Geometry check sheet. Reference: the model listing, model coordinates, mm. A direction names the side the tool comes from. Round coordinates to 2 decimals unless told otherwise and drop trailing zeros. Order: outer loops, then holes, each group sorted by start corner. A loop starts at its lowest first (then second) coordinate and runs counter-clockwise, first axis right, second up. Notation, with made-up numbers: (8.5, 58.5) - (40.5, 58.5) arc R28 cw to (40.5, 86.5) - close; hole circle Ø8 at (-37.5, -3.5). An arc over 180 degrees is marked (long way). Return JSON: item names as keys, results as strings. Group by question number.
Q1. Gauge pin test, flat ends, axial feed: pin 1 Ø8 at (x, y) = (69.28, -40) entering from -Z; pin 2 Ø10 at (x, y) = (11, 59) entering from -Z; pin 3 Ø3 at (x, z) = (-66.5, 2.5) entering from +Y; pin 4 Ø4 at (y, z) = (3.5, 6) entering from -X. Record the tip position at first contact, or that the pin passes through.
Q2. Tool access check on faces 4 (the flat face through (55.568, -10.884, 4.93)), 5 (the cylindrical face through (60.1, -26.1, 4.9)). Record the directions out of +Z, -Z, +X, -X, +Y, -Y that give a thin tool (end or side, any length) a straight path to the whole face; none if there is none.
Q3. Sectioned sample at C-C, the plane z = 5.5. Give the number of separate pieces and of enclosed holes in the cut face, then the cut area to 3 significant figures.
Q4. Sectioned sample at A-A, the plane x = 0. Record the cut outline in (y, z), then the cut area to 3 significant figures.
Q5. Draft check along Y on faces 1 (the cylindrical face through (-82.12, -47.76, 4.93)), 2 (the cylindrical face through (0, 65, 5)), 3 (the flat face through (37.933, -42.989, 4.93)). Enter one of: pulls with the +Y half, pulls with the -Y half, needs draft (parallel to the pull), parting line crosses it, or undercut.
Q6. Sectioned sample at B-B, the plane y = 80. Record the cut outline in (x, z), then the cut area to 3 significant figures.
Q7. Material ranges on line 1 along Y through (x, z) = (0, 4); line 2 along X through (y, z) = (-43.5, 1); line 3 along X through (y, z) = (-8, 8), recorded low to high.
Q8. Sectioned sample at D-D, the plane x = 43.5. Record the cut outline in (y, z), then the cut area to 3 significant figures.
```python
from build123d import *

# Parameters (mm, degrees)
SKETCH1_R           = 5
SKETCH1_R_2         = 10
BOSS_EXTRUDE1_DEPTH = 10


with BuildPart() as part:
    # Sketch1 → Boss-Extrude1 (new body)
    with BuildSketch(Plane.XY):
        with BuildLine():
            ThreePointArc((-33.454782287, 5.779804226), (-25.528470868, 14.738869527), (-21.732848432, 26.082789225))
            Line((-21.732848432, 26.082789225), (-14.888192275, 81.828040151))
            ThreePointArc((-14.888192275, 81.828040151), (0, 95), (14.888192275, 81.828040151))
            Line((14.888192275, 81.828040151), (21.732848432, 26.082789225))
            ThreePointArc((21.732848432, 26.082789225), (25.528470868, 14.738869527), (33.454782287, 5.779804226))
            Line((33.454782287, 5.779804226), (78.30925765, -28.020467349))
            ThreePointArc((78.30925765, -28.020467349), (82.27241336, -47.5), (63.421065375, -53.807572802))
            Line((63.421065375, -53.807572802), (11.721933855, -31.862593451))
            ThreePointArc((11.721933855, -31.862593451), (0, -29.477739055), (-11.721933855, -31.862593451))
            Line((-11.721933855, -31.862593451), (-63.421065375, -53.807572802))
            ThreePointArc((-63.421065375, -53.807572802), (-82.27241336, -47.5), (-78.30925765, -28.020467349))
            Line((-78.30925765, -28.020467349), (-33.454782287, 5.779804226))
        make_face()
        with Locations((-69.282032303, -40)):
            Circle(SKETCH1_R, mode=Mode.SUBTRACT)
        with Locations((69.282032303, -40)):
            Circle(SKETCH1_R, mode=Mode.SUBTRACT)
        with Locations((0, 80)):
            Circle(SKETCH1_R, mode=Mode.SUBTRACT)
        Circle(SKETCH1_R_2, mode=Mode.SUBTRACT)
        with BuildLine():
            ThreePointArc((-4.155876324, 65.587203881), (-7.469391302, 65.0809662), (-9.234294617, 62.231268956))
            Line((-9.234294617, 62.231268956), (-13.739592483, 25.538562373))
            ThreePointArc((-13.739592483, 25.538562373), (-11.624113874, 20.196928868), (-5.987935057, 19.082574086))
            ThreePointArc((-5.987935057, 19.082574086), (0, 20), (5.987935057, 19.082574086))
            ThreePointArc((5.987935057, 19.082574086), (11.624113874, 20.196928868), (13.739592483, 25.538562373))
            Line((13.739592483, 25.538562373), (9.234294617, 62.231268956))
            ThreePointArc((9.234294617, 62.231268956), (7.469391302, 65.0809662), (4.155876324, 65.587203881))
            ThreePointArc((4.155876324, 65.587203881), (0, 65), (-4.155876324, 65.587203881))
        make_face(mode=Mode.SUBTRACT)
        with BuildLine():
            ThreePointArc((58.878122886, -29.194507469), (60.096465683, -26.071800482), (58.511007134, -23.118500753))
            Line((58.511007134, -23.118500753), (28.986840033, -0.870445058))
            ThreePointArc((28.986840033, -0.870445058), (23.303110415, -0.031686522), (19.519961457, -4.355583168))
            ThreePointArc((19.519961457, -4.355583168), (17.320508076, -10), (13.5320264, -14.726990918))
            ThreePointArc((13.5320264, -14.726990918), (11.678996541, -20.165242346), (15.247247549, -24.668117315))
            Line((15.247247549, -24.668117315), (49.276712517, -39.112768202))
            ThreePointArc((49.276712517, -39.112768202), (52.627074381, -39.009165718), (54.722246562, -36.392696412))
            ThreePointArc((54.722246562, -36.392696412), (56.291651246, -32.5), (58.878122886, -29.194507469))
        make_face(mode=Mode.SUBTRACT)
        with BuildLine():
            ThreePointArc((-54.722246562, -36.392696412), (-52.627074381, -39.009165718), (-49.276712517, -39.112768202))
            Line((-49.276712517, -39.112768202), (-15.247247549, -24.668117315))
            ThreePointArc((-15.247247549, -24.668117315), (-11.678996541, -20.165242346), (-13.5320264, -14.726990918))
            ThreePointArc((-13.5320264, -14.726990918), (-17.320508076, -10), (-19.519961457, -4.355583168))
            ThreePointArc((-19.519961457, -4.355583168), (-23.303110415, -0.031686522), (-28.986840033, -0.870445058))
            Line((-28.986840033, -0.870445058), (-58.511007134, -23.118500753))
            ThreePointArc((-58.511007134, -23.118500753), (-60.096465683, -26.071800482), (-58.878122886, -29.194507469))
            ThreePointArc((-58.878122886, -29.194507469), (-56.291651246, -32.5), (-54.722246562, -36.392696412))
        make_face(mode=Mode.SUBTRACT)
    extrude(amount=BOSS_EXTRUDE1_DEPTH)


solid = part.part
```
Reply:
{
 "1": {"pin 1": "through", "pin 2": "z = 0", "pin 3": "y = -17.99", "pin 4": "x = -39.13"},
 "2": {"face 4": "+Z, -Z, +X, +Y", "face 5": "+Z, -Z"},
 "3": {"separate pieces": "1", "enclosed holes": "7", "area": "6,010 mm^2"},
 "4": {"outline": "(-29.48, 0) - (-10, 0) - (-10, 10) - (-29.48, 10) - close; (10, 0) - (20, 0) - (20, 10) - (10, 10) - close; (65, 0) - (75, 0) - (75, 10) - (65, 10) - close; (85, 0) - (95, 0) - (95, 10) - (85, 10) - close", "area": "495 mm^2"},
 "5": {"face 1": "parting line crosses it", "face 2": "undercut", "face 3": "pulls with the -Y half"},
 "6": {"outline": "(-15.11, 0) - (-5, 0) - (-5, 10) - (-15.11, 10) - close; (5, 0) - (15.11, 0) - (15.11, 10) - (5, 10) - close", "area": "202 mm^2"},
 "7": {"line 1": "-29.48 to -10, 10 to 20, 65 to 75, 85 to 95", "line 2": "-83.87 to -72.85, -65.71 to -39.14, 39.14 to 65.71, 72.85 to 83.87", "line 3": "-51.74 to -38.45, -18.33 to -6, 6 to 18.33, 38.45 to 51.74"},
 "8": {"outline": "(-45.35, 0) - (-36.66, 0) - (-36.66, 10) - (-45.35, 10) - close; (-11.81, 0) - (-1.79, 0) - (-1.79, 10) - (-11.81, 10) - close", "area": "187 mm^2"}
}
